Solid Edge part; units mm, degrees
sketch "Sketch1" plane through (0, 0, 0) normal (0, 0, 1) x (1, 0, 0)
  circle A0 centre (0, 0) radius 125
extrude "Protrusion1" add sketch "Sketch1" along normal blind 6
sketch "Sketch2" plane through (3.3435, -13.8996, 6) normal (0, 0, 1) x (1, 0, 0)
  line L0 (-13.3435, 116.8996) -> (6.6565, 116.8996)
  line L1 (6.6565, 116.8996) -> (6.6565, 122.8996)
  line L2 (6.6565, 122.8996) -> (-13.3435, 122.8996)
  line L3 (-13.3435, 122.8996) -> (-13.3435, 116.8996)
extrude "Cutout1" cut sketch "Sketch2" against normal through all
sketch "Sketch3" plane through (0.433, -2.3524, 6) normal (0, 0, 1) x (1, 0, 0)
  line L0 (-10.433, 119.3524) -> (9.567, 119.3524)
  line L1 (9.567, 119.3524) -> (9.567, 125.3524)
  line L2 (9.567, 125.3524) -> (-10.433, 125.3524)
  line L3 (-10.433, 125.3524) -> (-10.433, 119.3524)
extrude "Cutout2" cut sketch "Sketch3" against normal through all
pattern_circular "Pattern1" count 4 over 360 about axis through (0, 0, 6) along (0, 0, -1) of "Cutout2", "Cutout1"
properties material "Wood, Mahogany"
The model under review builds one solid part; all positions refer to its coordinate system, in mm. A direction names the side the tool comes from. Round coordinates to 2 decimals unless told otherwise and drop trailing zeros. Write each loop counter-clockwise with the first axis right and the second up, starting at its lowest first coordinate (ties: lowest second). Pieces come first, ordered by that corner, then holes.
(1) We need section C-C on z = 3.5. Give the number of separate pieces and of enclosed holes in the cut face, and give its area (3 significant figures).
(2) Insertion check: pin 1 (3 mm diameter, centred on x = 91.5, z = 3.5, fed in from +Y); pin 2 (3 mm diameter, centred on y = 1, z = 2, fed in from +X); pin 3 (1 mm diameter, centred on y = 97, z = 5, fed in from -X); pin 4 (3 mm diameter, centred on x = 104.5, z = 4, fed in from -Y). Each pin has a flat end and moves straight along its axis. Give the tip position at first contact, or say it passes through.
(3) We need section D-D on y = -85.5. Give the boundary of the cut face in (x, z), and give its area (3 significant figures).
(4) We need section A-A on x = 0. Give the boundary of the cut face in (y, z), and give its area (3 significant figures).
(5) Mouldability with a two-part tool opening along Y and no side actions: class faces 3 (the flat face through (-2, 2, 0)), 4 (the flat face through (10, 120, 3)), 5 (the flat face through (103, 0, 3)) as +Y half, -Y half, draft (parallel to the pull), parting line (faces both ways), or undercut.
(6) Wall thickness on L1, parallel to Y at x = 4.5, z = 3.8; L2, parallel to X at y = 6, z = 4.1; L3, parallel to Y at x = -113, z = 4.9: over which ranges is each line inside the solid? List them lowest first.
(7) Machinability: for faces 1 (the flat face through (0, -103, 3)), 2 (the flat face through (-2, 2, 6)), which of the approach directions +Z, -Z, +X, -X, +Y, -Y give a long, thin tool a straight path to every point of the face, cutting with its end or side? Answer none if there is none.
Findings below:
1. separate pieces: 1
1. enclosed holes: 8
1. area: 48,100 mm2
2. pin 1: stops at y = 86.75
2. pin 2: stops at x = 125
2. pin 3: stops at x = -79.45
2. pin 4: stops at y = -70.82
3. outline: (-91.19, 0) - (91.19, 0) - (91.19, 6) - (-91.19, 6) - close
3. area: 1,090 mm2
4. outline: (-125, 0) - (-123, 0) - (-123, 6) - (-125, 6) - close; (-117, 0) - (-109, 0) - (-109, 6) - (-117, 6) - close; (-103, 0) - (103, 0) - (103, 6) - (-103, 6) - close; (109, 0) - (117, 0) - (117, 6) - (109, 6) - close; (123, 0) - (125, 0) - (125, 6) - (123, 6) - close
4. area: 1,360 mm2
5. face 3: draft
5. face 4: undercut
5. face 5: undercut
6. L1: y = -124.92 to -123, -117 to -109, -103 to 103, 109 to 117, 123 to 124.92
6. L2: x = -124.86 to -123, -117 to -109, -103 to 103, 109 to 117, 123 to 124.86
6. L3: y = -53.44 to 53.44
7. face 1: +Z, -Z
7. face 2: +Z, +X, -X, +Y, -Y
